The model under review builds one solid part; all positions refer to its coordinate system, in mm. Face numbers are marked on the shaded views. A direction names the side the tool comes from. Round coordinates to 2 decimals unless told otherwise and drop trailing zeros. Write each loop counter-clockwise with the first axis right and the second up, starting at its lowest first coordinate (ties: lowest second). Pieces come first, ordered by that corner, then holes. Notation, with made-up numbers: (50.5, 53) - (82.5, 53) arc R13 cw to (82.5, 64) - close; hole circle Ø1 at (84, -27). An arc over 180 degrees is marked (long way). Use one line per item in the form item = value.
Autodesk Fusion 360 part; units mm, degrees
sketch "Szkic3" plane through (0, 0, 0) normal (0, 0, 1) x (1, 0, 0)
  line L0 (0, 0) -> (4, 0)
  line L1 (4, 0) -> (4, 10)
  line L2 (4, 10) -> (25, 10)
  line L3 (25, 10) -> (25, 14)
  line L4 (25, 14) -> (0, 14)
  line L5 (0, 14) -> (0, 0)
extrude "Wyciągnięcie proste3" add sketch "Szkic3" along normal blind 55
sketch "Szkic4" plane through (4, 0, 0) normal (1, 0, 0) x (0, 1, 0)
  line L0 (0, 0) -> (10, 0)
  line L1 (10, 0) -> (10, 55)
  line L2 (10, 55) -> (0, 55)
  line L3 (0, 55) -> (0, 0)
  circle A0 centre (6, 9) radius 1.75
  circle A1 centre (6, 47) radius 1.75
  dimension "d19" = 38
  dimension "d20" = 3.5
  dimension "d21" = 3.5
extrude "Wyciągnięcie proste4" cut sketch "Szkic4" against normal blind 4 contours A0 | A1
sketch "Szkic5" plane through (25, 0, 0) normal (1, 0, 0) x (0, 1, 0)
  line L0 (10, 0) -> (14, 0)
  line L1 (14, 0) -> (14, 55)
  line L2 (14, 55) -> (10, 55)
  line L3 (10, 55) -> (10, 0)
  line L4 (14, 55) -> (0, 55)
  line L5 (0, 55) -> (0, 15)
  line L6 (0, 15) -> (14, 15)
  line L7 (14, 15) -> (14, 55)
  line L8 (14, 3) -> (0, 3)
  line L9 (0, 3) -> (0, 0)
  line L10 (0, 0) -> (14, 0)
  line L11 (14, 0) -> (14, 3)
extrude "Wyciągnięcie proste5" cut sketch "Szkic5" against normal blind 37 contours L0 L1 L3 L8 L10 L11 | L3 L8 L9 L10 | L3 L4 L5 L6 | L1 L2 L3 L4 L6 L7
sketch "Szkic6" plane through (0, 10, 0) normal (0, -1, 0) x (1, 0, 0)
  line L0 (25, 15) -> (4, 15)
  line L1 (4, 15) -> (4, 3)
  line L2 (4, 3) -> (25, 3)
  line L3 (25, 3) -> (25, 15)
  line L4 (25, 15) -> (15, 15)
  line L5 (15, 15) -> (15, 3)
  line L6 (15, 3) -> (25, 3)
  line L7 (25, 3) -> (25, 15)
  circle A0 centre (9, 9) radius 2.5
  dimension "d26" = 5
extrude "Wyciągnięcie proste6" cut sketch "Szkic6" against normal blind 4 contours L0 L2 L3 L4 L5 L6 L7 | A0
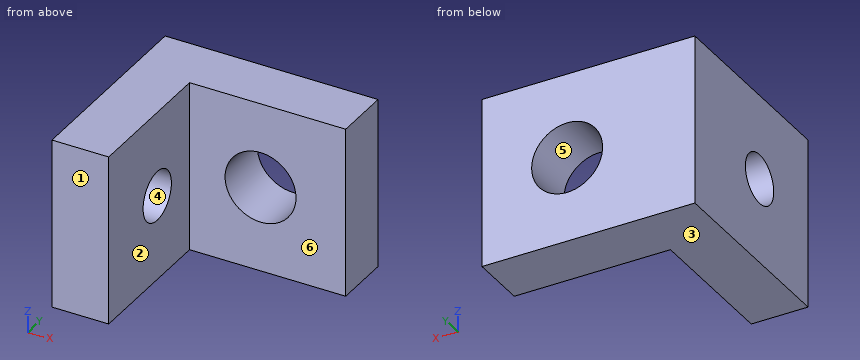
(1) The part is to be moulded in two halves that separate along Z. For the marked faces 3, 4, 5 and 6, say which applies: +Z half, -Z half, draft (parallel to the pull), parting line (faces both ways), or undercut.
Geometry results:
face_3 = -Z half
face_4 = undercut
face_5 = undercut
face_6 = draft
(2) Insertion check: P1, Ø6.5, axis at x = 9, z = 9, coming from the -Y side; P2, Ø3, axis at y = 9, z = 6, coming from the +X side; P3, Ø5, axis at y = 5, z = 9.5, coming from the +X side; P4, Ø2, axis at y = 6, z = 9, coming from the -X side. Each pin has a flat end and moves straight along its axis. Give the tip position at first contact, or say it passes through.
Geometry results:
P1 = 10
P2 = 15
P3 = 4
P4 = through
(3) To check wall thickness, follow L1, parallel to Z at x = 0.9, y = 6; L2, parallel to Z at x = 9, y = 13; L3, parallel to X at y = 2.25, z = 5.5. State the ranges of each line that lie inside material, in increasing order.
Geometry results:
L1 = 3 to 7.25, 10.75 to 15
L2 = 3 to 6.5, 11.5 to 15
L3 = 0 to 4
(4) Add section B-B on y = 6. Write out the cut boundary in (x, z), then the cut area to 3 significant figures.
Geometry results:
outline = (0, 3) - (4, 3) - (4, 7.25) - (0, 7.25) - close; (0, 10.75) - (4, 10.75) - (4, 15) - (0, 15) - close
area = 34.0 mm2
(5) Add section D-D on y = 11. Write out the cut boundary in (x, z), then the cut area to 3 significant figures.
Geometry results:
outline = (0, 3) - (15, 3) - (15, 15) - (0, 15) - close; hole circle Ø5 at (9, 9)
area = 160 mm2
(6) Add section A-A on x = 7. Write out the cut boundary in (y, z), then the cut area to 3 significant figures.
Geometry results:
outline = (10, 3) - (14, 3) - (14, 7.5) - (10, 7.5) - close; (10, 10.5) - (14, 10.5) - (14, 15) - (10, 15) - close
area = 36.0 mm2
(7) Machinability: for the marked faces 1 and 2, which of the approach directions +Z, -Z, +X, -X, +Y, -Y give a long, thin tool a straight path to every point of the face, cutting with its end or side? Answer none if there is none.
Geometry results:
face_1 = +Z, -Z, +X, -X, -Y
face_2 = +Z, -Z, +X, -Y
(8) Add section C-C on z = 9. Write out the cut boundary in (x, y).
Geometry results:
outline = (0, 0) - (4, 0) - (4, 4.25) - (0, 4.25) - close; (0, 7.75) - (4, 7.75) - (4, 10) - (6.5, 10) - (6.5, 14) - (0, 14) - close; (11.5, 10) - (15, 10) - (15, 14) - (11.5, 14) - close
